```python
from build123d import *

# Parameters (mm, degrees)
SKETCH1_W           = 28
SKETCH1_H           = 16
BOSS_EXTRUDE1_DEPTH = 10
SKETCH2_W           = 2
SKETCH2_H           = 25
BOSS_EXTRUDE2_DEPTH = 0.5
SKETCH3_R           = 1.5
CUT_EXTRUDE1_DEPTH  = 10


with BuildPart() as part:
    # Sketch1 → Boss-Extrude1 (new body)
    with BuildSketch(Plane(origin=(0, 0, 0), x_dir=(1, 0, 0), z_dir=(0, 1, 0))):
        Rectangle(SKETCH1_W, SKETCH1_H)
    extrude(amount=BOSS_EXTRUDE1_DEPTH)

    # Sketch2 → Boss-Extrude2 (add, symmetric)
    with BuildSketch(Plane(origin=(6.964101615, 0, 12.062177826), x_dir=(0, -1, 0), z_dir=(0.5, 0, 0.866025404))):
        with Locations((-5, -4.375644347)):
            Rectangle(SKETCH2_W, SKETCH2_H)
    extrude(amount=BOSS_EXTRUDE2_DEPTH, both=True)

    # Sketch3 → Cut-Extrude1 (cut)
    with BuildSketch(Plane(origin=(0, 10, 0), x_dir=(1, 0, 0), z_dir=(0, 1, 0))):
        with Locations((-11, 5)):
            Circle(SKETCH3_R)
    extrude(amount=-CUT_EXTRUDE1_DEPTH, mode=Mode.SUBTRACT)


solid = part.part
```
Here's how the part is built. I have some questions about the finished solid (model axes, mm). A direction names the side the tool comes from. Round coordinates to 2 decimals unless told otherwise and drop trailing zeros. Order: outer loops, then holes, each group sorted by start corner. A loop starts at its lowest first (then second) coordinate and runs counter-clockwise, first axis right, second up. Notation, with made-up numbers: (52, 77) -> (85, 77) arc R28 ccw to (85, 102) -> close; hole circle Ø1 at (62, 63.5). An arc over 180 degrees is marked (long way). Use a Markdown table: item, result. Add a question column.
(1) Suppose I cut it at C-C, the plane y = 5. Please give me the cut outline in (x, z).
(2) For pin 1 Ø6.5 at (x, z) = (7.5, 13) entering from +Y; pin 2 Ø1.5 at (y, z) = (6, 2) entering from +X; pin 3 Ø6 at (x, y) = (3, 5) entering from +Z, each with a flat end and sliding along its axis, tell me the tip position at first contact or that it passes through.
(3) Suppose I cut it at B-B, the plane x = -11. Please give me the cut outline in (y, z), and give its area (3 significant figures).
(4) Suppose I cut it at A-A, the plane z = -5. Please give me the cut outline in (x, y), and give its area (3 significant figures).
(5) I need wall thicknesses on line 1 along Z through (x, y) = (-11, 3); line 2 along X through (y, z) = (4.25, -5); line 3 along X through (y, z) = (1.75, 4.25). Which ranges of each line are inside material? Lowest first, please.
(6) Suppose I cut it at D-D, the plane y = 8.75. Please give me the cut outline in (x, z).
(7) For faces 1 (the face through (0, 0, 0)), 2 (the face through (3, 4, 14)), which set-ups out of +Z, -Z, +X, -X, +Y, -Y let a thin tool reach every point of the face, with its end or its side?
(8) If we mould it in two halves opening along Z, with no side actions, what happens to faces 3 (the face through (3, 6, 14)), 4 (the face through (3.576, 5.014, 14.596)), 5 (the face through (-12.5, 5.07, -5.07)), 6 (the face through (2.696, 5.014, 13.949))? For each: released by +Z, released by -Z, zero draft, split by the parting line, or undercut.
Verdict:
| question | item | result |
|---|---|---|
| 1 | outline | (-14, -8) -> (14, -8) -> (14, 8) -> (14.25, 8.43) -> (-7.4, 20.93) -> (-7.9, 20.07) -> (13, 8) -> (-14, 8) -> close; hole circle Ø3 at (-11, -5) |
| 2 | pin 1 | y = 6 |
| 2 | pin 2 | x = 14 |
| 2 | pin 3 | z = 16.66 |
| 3 | outline | (0, -8) -> (10, -8) -> (10, -6.5) -> (0, -6.5) -> close; (0, -3.5) -> (10, -3.5) -> (10, 8) -> (0, 8) -> close |
| 3 | area | 130 mm2 |
| 4 | outline | (-14, 0) -> (-12.5, 0) -> (-12.5, 10) -> (-14, 10) -> close; (-9.5, 0) -> (14, 0) -> (14, 10) -> (-9.5, 10) -> close |
| 4 | area | 250 mm2 |
| 5 | line 1 | -8 to -6.5, -3.5 to 8 |
| 5 | line 2 | -14 to -12.5, -9.5 to 14 |
| 5 | line 3 | -14 to 14 |
| 6 | outline | (-14, -8) -> (14, -8) -> (14, 8) -> (-14, 8) -> close; hole circle Ø3 at (-11, -5) |
| 7 | face 1 | +Z, -Z, +X, -X, -Y |
| 7 | face 2 | +Z, +X, -X, -Y |
| 8 | face 3 | zero draft |
| 8 | face 4 | released by +Z |
| 8 | face 5 | undercut |
| 8 | face 6 | undercut |
